```python
from build123d import *

# Parameters (mm, degrees)
SKETCH1_R           = 2.0193
BOSS_EXTRUDE1_DEPTH = 50.00625
SKETCH2_OUTSIDE_W   = 36.1
SKETCH2_OUTSIDE_H   = 35.05
SKETCH2_OUTSIDE_R   = 6.35
CUT_EXTRUDE2_DEPTH  = 7.9375


with BuildPart() as part:
    # Sketch1 → Boss-Extrude1 (new, symmetric)
    with BuildSketch(Plane.XY):
        with BuildLine():
            ThreePointArc((4.181770846, 5.456960429), (3.437499983, 5.953924622), (2.634980936, 6.35))
            Line((2.634980936, 6.35), (-2.634980936, 6.35))
            ThreePointArc((-2.634980936, 6.35), (-3.437499983, 5.953924622), (-4.181770846, 5.456960429))
            Line((-4.181770846, 5.456960429), (-6.816751782, 0.893039571))
            ThreePointArc((-6.816751782, 0.893039571), (-6.874999966, 0), (-6.816751782, -0.893039571))
            Line((-6.816751782, -0.893039571), (-4.181770846, -5.456960429))
            ThreePointArc((-4.181770846, -5.456960429), (-3.437499983, -5.953924622), (-2.634980936, -6.35))
            Line((-2.634980936, -6.35), (2.634980936, -6.35))
            ThreePointArc((2.634980936, -6.35), (3.437499983, -5.953924622), (4.181770846, -5.456960429))
            Line((4.181770846, -5.456960429), (6.816751782, -0.893039571))
            ThreePointArc((6.816751782, -0.893039571), (6.860422465, -0.447468582), (6.874999966, 0))
            ThreePointArc((6.874999966, 0), (6.860422465, 0.447468582), (6.816751782, 0.893039571))
            Line((6.816751782, 0.893039571), (4.181770846, 5.456960429))
        make_face()
        with Locations(Location((0, 0, 0), (0, 0, 180))):
            Circle(SKETCH1_R, mode=Mode.SUBTRACT)
    extrude(amount=BOSS_EXTRUDE1_DEPTH, both=True)

    # Sketch2 outside → Cut-Extrude2 (cut)
    with BuildSketch(Plane.XY.offset(50.00625)):
        Rectangle(SKETCH2_OUTSIDE_W, SKETCH2_OUTSIDE_H)
        Circle(SKETCH2_OUTSIDE_R, mode=Mode.SUBTRACT)
    extrude(amount=-CUT_EXTRUDE2_DEPTH, mode=Mode.SUBTRACT)


solid = part.part
```
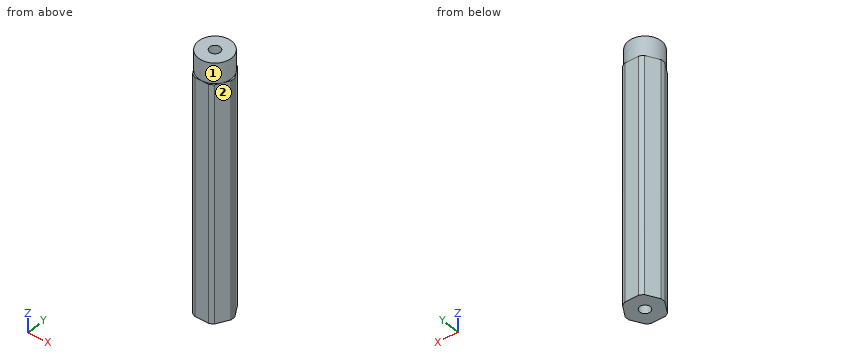
Part model, mm, in its own coordinate system. Face numbers are marked on the shaded views. A direction names the side the tool comes from. Round coordinates to 2 decimals unless told otherwise and drop trailing zeros. Loops run counter-clockwise (first coordinate to the right, second up) from the corner with the lowest first, then second, coordinate; pieces in that order, holes last. Notation, with made-up numbers: (-11.75, 45.5) -> (20.25, 45.5) arc R19 cw to (20.25, 72.5) -> close; hole circle Ø2 at (78.25, 34). An arc over 180 degrees is marked (long way). Use a Markdown table: item, result.
1) Drop flat-ended pins along their axis: pin 1 Ø6 at (y, z) = (-4, -6) entering from -X (3 decimals); pin 2 Ø5 at (y, z) = (3.5, -0.5) entering from +X (3 decimals); pin 3 Ø1.5 at (y, z) = (-2, 38) entering from +X. Give the stop position or say it passes through.
The answers:
| item | result |
|---|---|
| pin 1 | stops at x = -6.755 |
| pin 2 | stops at x = 6.755 |
| pin 3 | stops at x = 6.61 |
2) Cut at A-A, the plane z = 6.5. List the corners of the cut face in (x, y) (3 decimals).
The answers:
| item | result |
|---|---|
| outline | (-6.817, -0.893) -> (-4.182, -5.457) arc R6.875 ccw to (-2.635, -6.35) -> (2.635, -6.35) arc R6.875 ccw to (4.182, -5.457) -> (6.817, -0.893) arc R6.875 ccw to (6.817, 0.893) -> (4.182, 5.457) arc R6.875 ccw to (2.635, 6.35) -> (-2.635, 6.35) arc R6.875 ccw to (-4.182, 5.457) -> (-6.817, 0.893) arc R6.875 ccw to start; hole circle Ø4.039 at (0, 0) |
3) Tool access for the marked faces 1 and 2: list every direction of +Z, -Z, +X, -X, +Y, -Y with a clear straight run to the whole face (end or side of a thin tool).
The answers:
| item | result |
|---|---|
| face 1 | +Z |
| face 2 | +Z, -Z, +X, -Y |
4) Probe line 1 (Y direction, x = 0, z = 13); line 2 (Y direction, x = 1.5, z = 31); line 3 (Y direction, x = -5.5, z = 25). List the from-to ranges inside material, lowest first. Write a range as [from, to].
The answers:
| item | result |
|---|---|
| line 1 | y = [-6.35, -2.02], [2.02, 6.35] |
| line 2 | y = [-6.35, -1.35], [1.35, 6.35] |
| line 3 | y = [-3.17, 3.17] |
